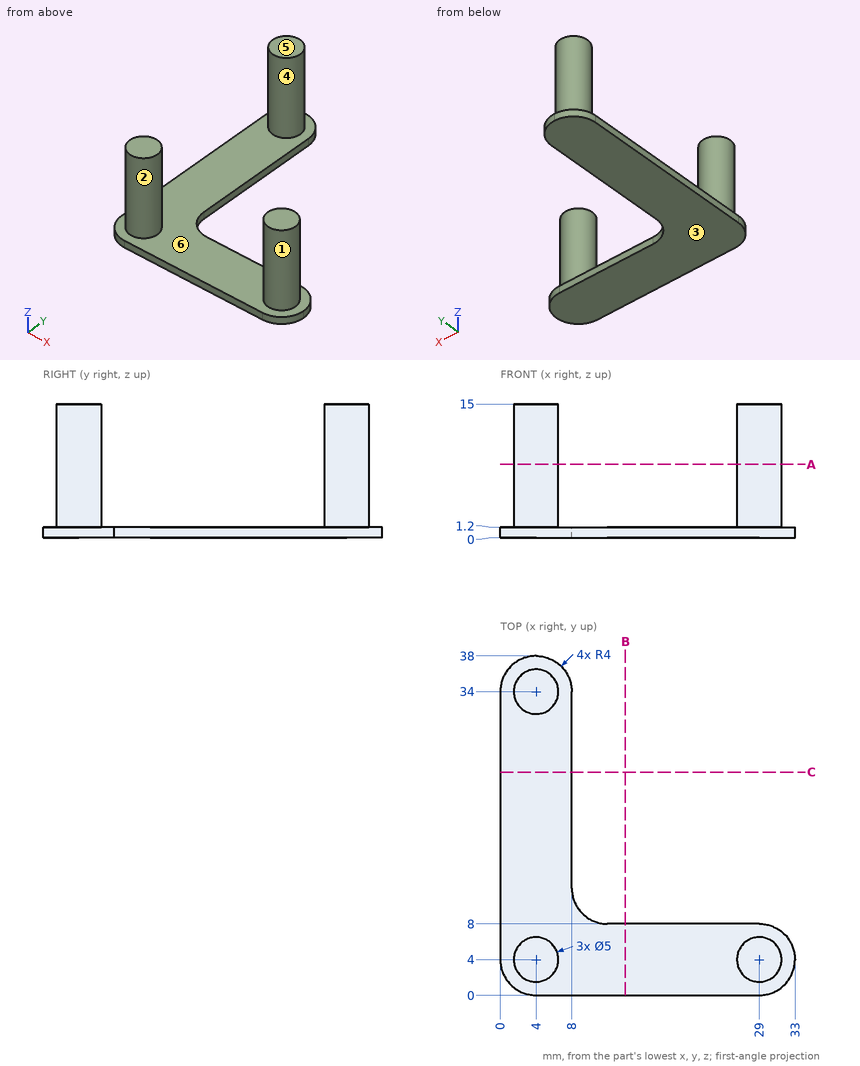
Here's the drawing with two shaded views (mm, measured from the low corner). I have some questions. A direction names the side the tool comes from. Give positions to 0.01 mm unless a question says otherwise; leave off trailing zeros. Write each loop counter-clockwise with the first axis right and the second up, starting at its lowest first coordinate (ties: lowest second). Pieces come first, ordered by that corner, then holes. Notation, with made-up numbers: (-36, 26) -> (-26, 26) arc R13 ccw to (-26, 37) -> close; hole circle Ø6 at (73.5, -3). An arc over 180 degrees is marked (long way). Answer as a JSON object with one key per item and string values. Group by question number.
Item 1: We'd pull the mould along X, two halves only. Please class the marked faces 1, 2, 3 and 4: +X half, -X half, draft (parallel to the pull), parting line (faces both ways), or undercut.
Item 2: Please list where these lines run through material, in increasing order: line 1 (X direction, y = 30, z = 1); line 2 (X direction, y = 5, z = 4.75). Write a range as [from, to].
Item 3: I'm going to push flat-ended pins straight in: P1, Ø1.5, axis at x = 15, z = 2, coming from the +Y side; P2, Ø1.3, axis at y = 23.5, z = 0.5, coming from the +X side; P3, Ø6, axis at x = 18, z = 3.5, coming from the +Y side. Where does each tip first touch, or does it pass through?
Item 4: Suppose I cut it at A-A (z = 8.25). Please give me the cut outline in (x, y), plus the area to 3 significant figures.
Item 5: For the marked faces 5 and 6, which set-ups out of +Z, -Z, +X, -X, +Y, -Y let a thin tool reach every point of the face, with its end or its side?
Item 6: Suppose I cut it at B-B (x = 14). Please give me the cut outline in (y, z).
Findings:
{
 "1": {"face 1": "undercut", "face 2": "undercut", "face 3": "draft", "face 4": "parting line"},
 "2": {"line 1": "x = [0, 8]", "line 2": "x = [1.71, 6.29], [26.71, 31.29]"},
 "3": {"P1": "passes through", "P2": "stops at x = 8", "P3": "stops at y = 8"},
 "4": {"outline": "circle Ø5 at (4, 4); circle Ø5 at (4, 34); circle Ø5 at (29, 4)", "area": "58.9 mm²"},
 "5": {"face 5": "+Z, +X, -X, +Y, -Y", "face 6": "+Z"},
 "6": {"outline": "(0, 0) -> (8, 0) -> (8, 1.2) -> (0, 1.2) -> close"}
}
